The model under review builds one solid part; all positions refer to its coordinate system, in mm. Give positions to 0.01 mm unless a question says otherwise; leave off trailing zeros. Write each loop counter-clockwise with the first axis right and the second up, starting at its lowest first coordinate (ties: lowest second). Pieces come first, ordered by that corner, then holes. Notation, with made-up numbers: (27, 75) -> (39, 75) arc R19 cw to (39, 84) -> close; hole circle Ø11 at (88, -14). An arc over 180 degrees is marked (long way). Use CSV: the item, a comma, the result in double quotes.
```python
from build123d import *

# Parameters (mm, degrees)
F0_R     = 9.525
F0_R_2   = 4.7625
F0_R_3   = 6.35
F1_DEPTH = 3.175


with BuildPart() as f1:
    # F0 (on Front) → F1 (new body)
    with BuildSketch(Plane.XZ):
        with BuildLine():
            Line((25.045655, -440.212115), (74.606246, -10.776475))
            Line((74.606246, -10.776475), (-73.023894, -10.329813))
            Line((-73.023894, -10.329813), (-27.010583, -440.160007))
            ThreePointArc((-27.010583, -440.160007), (-24.941095, -444.207157), (-20.696658, -445.834102))
            Line((-20.696658, -445.834102), (-20.053171, -445.834102))
            Line((-20.053171, -445.834102), (-20.053171, -414.084102))
            ThreePointArc((-20.053171, -414.084102), (-1.003171, -395.034102), (18.046829, -414.084102))
            Line((18.046829, -414.084102), (18.046829, -445.834102))
            Line((18.046829, -445.834102), (18.737525, -445.834102))
            ThreePointArc((18.737525, -445.834102), (22.962429, -444.224639), (25.045655, -440.212115))
        make_face()
        with BuildLine():
            Line((-6.32504, -306.535779), (-24.381244, -137.864985))
            Line((-24.381244, -137.864985), (-33.503104, -52.653751))
            Line((-33.503104, -52.653751), (-34.255227, -45.627845))
            Line((-34.255227, -45.627845), (-15.339314, -110.402874))
            ThreePointArc((-15.339314, -110.402874), (-0.09162, -90.077848), (15.132605, -110.420459))
            Line((15.132605, -110.420459), (34.13484, -45.627845))
            Line((34.13484, -45.627845), (33.38561, -52.651402))
            Line((33.38561, -52.651402), (24.04055, -140.255525))
            Line((24.04055, -140.255525), (6.303062, -306.533431))
            ThreePointArc((6.303062, -306.533431), (-0.009934, -312.209874), (-6.32504, -306.535779))
        make_face(mode=Mode.SUBTRACT)
        with BuildLine():
            ThreePointArc((283.113571, 171.791383), (283.396441, 178.307404), (277.787406, 181.635659))
            Line((277.787406, 181.635659), (123.630658, 181.051308))
            ThreePointArc((123.630658, 181.051308), (123.618623, 181.051274), (123.606587, 181.051262))
            Line((123.606587, 181.051262), (80.956246, 181.051262))
            ThreePointArc((80.956246, 181.051262), (76.466118, 182.911134), (74.606246, 187.401262))
            Line((74.606246, 187.401262), (74.606246, 224.240675))
            ThreePointArc((74.606246, 224.240675), (76.46202, 228.726701), (80.94465, 230.590665))
            Line((80.94465, 230.590665), (123.407974, 230.668213))
            ThreePointArc((123.407974, 230.668213), (127.890604, 232.532177), (129.746377, 237.018203))
            Line((129.746377, 237.018203), (129.746377, 332.519098))
            Line((129.746377, 332.519098), (129.746377, 380.139775))
            ThreePointArc((129.746377, 380.139775), (127.886505, 384.629903), (123.396377, 386.489775))
            Line((123.396377, 386.489775), (-110.029623, 386.489775))
            Line((-110.029623, 386.489775), (-148.129623, 386.489775))
            ThreePointArc((-148.129623, 386.489775), (-152.619751, 384.629903), (-154.479623, 380.139775))
            Line((-154.479623, 380.139775), (-154.479623, 236.828389))
            ThreePointArc((-154.479623, 236.828389), (-152.619751, 232.338261), (-148.129623, 230.478389))
            Line((-148.129623, 230.478389), (-110.029623, 230.478389))
            Line((-110.029623, 230.478389), (-84.143754, 230.478389))
            ThreePointArc((-84.143754, 230.478389), (-79.653625, 228.618517), (-77.793754, 224.128389))
            Line((-77.793754, 224.128389), (-77.793754, 186.028389))
            ThreePointArc((-77.793754, 186.028389), (-79.653625, 181.538261), (-84.143754, 179.678389))
            Line((-84.143754, 179.678389), (-116.379623, 179.678389))
            Line((-116.379623, 179.678389), (-234.864242, 179.692387))
            Line((-234.864242, 179.692387), (-271.483406, 179.553577))
            ThreePointArc((-271.483406, 179.553577), (-277.502393, 175.153997), (-275.191033, 168.065829))
            ThreePointArc((-275.191033, 168.065829), (-268.123306, 164.463433), (-260.288993, 163.217018))
            ThreePointArc((-260.288993, 163.217018), (-157.167464, 117.40772), (-121.820214, 10.24843))
            ThreePointArc((-121.820214, 10.24843), (-117.099081, -4.08894), (-103.313719, -10.238169))
            Line((-103.313719, -10.238169), (-73.023894, -10.329813))
            Line((-73.023894, -10.329813), (74.606246, -10.776475))
            Line((74.606246, -10.776475), (103.112156, -10.862721))
            ThreePointArc((103.112156, -10.862721), (118.963009, -3.924558), (124.520268, 12.461549))
            ThreePointArc((124.520268, 12.461549), (160.203696, 116.857109), (261.585693, 160.370679))
            ThreePointArc((261.585693, 160.370679), (273.808739, 163.330633), (283.113571, 171.791383))
        make_face()
        with BuildLine():
            Line((-103.257282, 154.791078), (-103.257282, 39.461342))
            ThreePointArc((-103.257282, 39.461342), (-124.759996, 104.793935), (-171.993459, 154.791078))
            Line((-171.993459, 154.791078), (-103.257282, 154.791078))
        make_face(mode=Mode.SUBTRACT)
        with Locations((0, 90.778389)):
            Circle(F0_R, mode=Mode.SUBTRACT)
        with Locations((0, 154.278389)):
            Circle(F0_R, mode=Mode.SUBTRACT)
        with Locations((-135.429623, 259.494098)):
            Circle(F0_R_2, mode=Mode.SUBTRACT)
        with Locations((-90.424, 259.494098)):
            Circle(F0_R_3, mode=Mode.SUBTRACT)
        with Locations((-135.429623, 354.744098)):
            Circle(F0_R_2, mode=Mode.SUBTRACT)
        with Locations((-90.424, 354.744098)):
            Circle(F0_R_3, mode=Mode.SUBTRACT)
        with BuildLine():
            Line((103.051167, 44.596632), (103.176985, 155.552762))
            Line((103.176985, 155.552762), (168.951373, 155.552762))
            ThreePointArc((168.951373, 155.552762), (124.191688, 107.754936), (103.176985, 45.73523))
            ThreePointArc((103.176985, 45.73523), (103.113024, 45.166047), (103.051167, 44.596632))
        make_face(mode=Mode.SUBTRACT)
        with BuildLine():
            ThreePointArc((74.500873, 184.222761), (74.606246, 184.226262), (74.71162, 184.222761))
            Line((74.71162, 184.222761), (74.500873, 184.222761))
        make_face(mode=Mode.SUBTRACT)
        with Locations((104.902, 259.494098)):
            Circle(F0_R_3, mode=Mode.SUBTRACT)
        with Locations((104.902, 354.744098)):
            Circle(F0_R_3, mode=Mode.SUBTRACT)
    extrude(amount=F1_DEPTH)


solid = f1.part
```
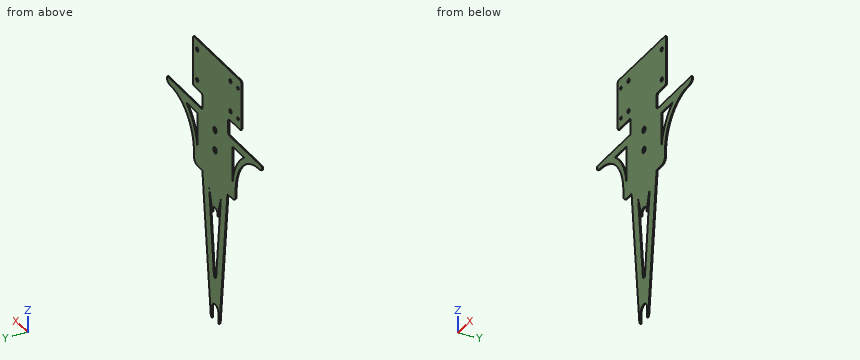
Q1. Consider section A-A (z = -214.5). Write out the cut boundary in (x, y) (3 decimals).
Derived:
outline,"(-51.167, -3.175) -> (-16.177, -3.175) -> (-16.177, 0) -> (-51.167, 0) -> close; (16.121, -3.175) -> (51.095, -3.175) -> (51.095, 0) -> (16.121, 0) -> close"
Q2. Insertion check: pin 1 (6 mm diameter, centred on x = 60.5, z = -20.5, fed in from +Y); pin 2 (1 mm diameter, centred on y = -1.5, z = 198, fed in from -X); pin 3 (1.6 mm diameter, centred on y = -2, z = 89, fed in from -X); pin 4 (1 mm diameter, centred on y = -1.5, z = 298.5, fed in from +X). Each pin has a flat end and moves straight along its axis. Give the tip position at first contact, or say it passes through.
Derived:
pin 1,"stops at y = 0"
pin 2,"stops at x = -77.79"
pin 3,"stops at x = -137.7"
pin 4,"stops at x = 129.75"
Q3. Consider section B-B (x = 145). Write out the cut boundary in (y, z) (3 decimals).
Derived:
outline,"(-3.175, 97.083) -> (0, 97.083) -> (0, 135.085) -> (-3.175, 135.085) -> close; (-3.175, 155.553) -> (0, 155.553) -> (0, 181.132) -> (-3.175, 181.132) -> close"
Q4. Consider section D-D (z = 295). Write out the cut boundary in (x, y) (3 decimals), then the cut area to 3 significant figures.
Derived:
outline,"(-154.48, -3.175) -> (129.746, -3.175) -> (129.746, 0) -> (-154.48, 0) -> close"
area,"902 mm2"
Q5. To check wall thickness, follow probe 1 along Z at (x, y) = (0, -1.2); probe 2 along Z at (x, y) = (-215, -2.5); probe 3 along X at (y, z) = (-0.25, 147). State the ranges of each line that lie inside material, in increasing order.
Derived:
probe 1,"z = -395.06 to -312.21, -90.08 to 81.25, 100.3 to 144.75, 163.8 to 386.49"
probe 2,"z = 155.6 to 179.69"
probe 3,"x = -195.2 to -161.44, -103.26 to -6.14, 6.14 to 103.17, 157.72 to 201.07"
